from build123d import *

# Parameters (mm, degrees)
SKETCH1_W           = 190
SKETCH1_H           = 3
EXTRUDE_THIN1_DEPTH = 120
BOSS_EXTRUDE1_DEPTH = 3
FILLET2_R           = 10
SKETCH4_R           = 7
SKETCH4_R_2         = 10
CUT_EXTRUDE1_DEPTH  = 3


with BuildPart() as part:
    # Sketch1 → Extrude-Thin1 (new body)
    with BuildSketch(Plane.XY):
        with Locations((95, -1.5)):
            Rectangle(SKETCH1_W, SKETCH1_H)
    extrude(amount=EXTRUDE_THIN1_DEPTH)

    # Sketch3 → Boss-Extrude1 (add)
    with BuildSketch(Plane(origin=(0, 0, 0), x_dir=(-1, 0, 0), z_dir=(0, 0, -1))):
        Polygon((-190, 0), (-190, 100), (110, 220), (110, 0), (110, -3), (-190, -3), align=None)
    extrude(amount=BOSS_EXTRUDE1_DEPTH)

    # Fillet2
    fillet2_edges = [part.edges().sort_by_distance(p)[0] for p in [
        (0, -1.5, 120),
        (-110, -3, -1.5),
        (-110, 220, -1.5),
        (190, 100, -1.5),
        (0, -1.5, 0),
        (190, -1.5, 120),
    ]]
    fillet(fillet2_edges, radius=FILLET2_R)

    # Sketch4 → Cut-Extrude1 (cut)
    with BuildSketch(Plane(origin=(0, 0, -3), x_dir=(-1, 0, 0), z_dir=(0, 0, -1))):
        with Locations((-42.372187551, 66.2)):
            Circle(SKETCH4_R)
        with Locations((19.981641522, 66.2)):
            Circle(SKETCH4_R)
        with Locations((-11.195273015, 120.2)):
            Circle(SKETCH4_R)
        with Locations((-11.195273015, 84.2)):
            Circle(SKETCH4_R_2)
    extrude(amount=-CUT_EXTRUDE1_DEPTH, mode=Mode.SUBTRACT)


solid = part.part
Check sheet for the modelled part. Datum: model origin and axes. Units: mm. Give positions to 0.01 mm unless a question says otherwise; leave off trailing zeros. Loops run counter-clockwise (first coordinate to the right, second up) from the corner with the lowest first, then second, coordinate; pieces in that order, holes last. Notation, with made-up numbers: M -29,24.5 L -12,24.5 A14 cw -12,49.5 Z; hole C 59.5,36.5 d7. An arc over 180 degrees is marked long. Answer as a JSON object with one key per item and string values. Group by question number.
Q1. Cross-section at B-B on x = 147. Record the cut outline in (y, z).
Q2. Go/stop test with flat-tipped pins: P1, Ø1.5, axis at x = 66, z = 31.5, coming from the +Y side; P2, Ø0.9, axis at y = -2, z = 70.5, coming from the -X side. Record where each tip stops, or that it passes through.
Q3. Release check for a two-part mould opening along Y. For faces 1 (the flat face through (190, -1, 29)), 2 (the flat face through (89, 0, 59)), 3 (the flat face through (107, -3, 59)), 4 (the cylindrical face through (13.363, 74.438, -1.521)) record: released by +Y, released by -Y, zero draft, split by the parting line, or undercut.
Q4. Cross-section at A-A on y = 84.2. Record the cut outline in (x, z).
Q5. Cross-section at C-C on y = 120.2. Record the cut outline in (x, z), then the cut area to 4 significant figures.
Q6. Cross-section at D-D on z = 40.5. Record the cut outline in (x, y), then the cut area to 3 significant figures.
Q7. Material ranges on line 1 along Z through (x, y) = (-6.5, 58.5), recorded low to high. Write a range as [from, to].
Evaluation:
{
 "1": {"outline": "M -3,-3 L 117.2,-3 L 117.2,0 L 0,0 L 0,120 L -3,120 Z"},
 "2": {"P1": "stops at y = 0", "P2": "stops at x = 0"},
 "3": {"face 1": "zero draft", "face 2": "released by +Y", "face 3": "released by -Y", "face 4": "undercut"},
 "4": {"outline": "M -110,-3 L 1.2,-3 L 1.2,0 L -110,0 Z; M 21.2,-3 L 190,-3 L 190,0 L 21.2,0 Z"},
 "5": {"outline": "M -110,-3 L 4.2,-3 L 4.2,0 L -110,0 Z; M 18.2,-3 L 139.5,-3 L 139.5,0 L 18.2,0 Z", "area": "706.5 mm2"},
 "6": {"outline": "M 0,-3 L 190,-3 L 190,0 L 0,0 Z", "area": "570 mm2"},
 "7": {"line 1": "z = [-3, 0]"}
}
